The model under review builds one solid part; all positions refer to its coordinate system, in mm. A direction names the side the tool comes from. Round coordinates to 2 decimals unless told otherwise and drop trailing zeros. Write each loop counter-clockwise with the first axis right and the second up, starting at its lowest first coordinate (ties: lowest second). Pieces come first, ordered by that corner, then holes. Notation, with made-up numbers: M 12,-9 L 29,-9 A21 cw 29,23 Z; hole C -31.5,-4.5 d2. An arc over 180 degrees is marked long. Write item = value, one per line. Start each with the question number.
Item 1: Tool access review of faces 1 (the flat face through (-62, 40, -1)), 2 (the flat face through (-88, 20, 1)): name each direction out of +Z, -Z, +X, -X, +Y, -Y from which nothing blocks a thin tool from reaching the whole face with its end or side.
Item 2: The part is to be moulded in two halves that separate along Z. For faces 3 (the flat face through (28.5, 20, -136)), 4 (the flat face through (-205, 20, 2)), say which applies: +Z half, -Z half, draft (parallel to the pull), parting line (faces both ways), or undercut.
Item 3: Take a section at A-A, the plane x = 74. Give the boundary of the cut face in (y, z).
Item 4: Take a section at B-B, the plane z = 97.5. Give the boundary of the cut face in (x, y).
Item 5: Take a section at D-D, the plane x = 14. Give the boundary of the cut face in (y, z).
Item 6: Take a section at C-C, the plane y = 29. Give the boundary of the cut face in (x, z).
Item 7: To check wall thickness, follow line 1 along X through (y, z) = (16.5, -73); line 2 along Z through (x, y) = (-3.5, 17); line 3 along Z through (x, y) = (-116, 22). State the ranges of each line that lie inside material, in increasing order.
from build123d import *

# Parameters (mm, degrees)
SKETCH1_W           = 410
SKETCH1_H           = 341
BOSS_EXTRUDE1_DEPTH = 40


with BuildPart() as part:
    # Sketch1 → Boss-Extrude1 (new body)
    with BuildSketch(Plane(origin=(0, 0, 0), x_dir=(1, 0, 0), z_dir=(0, 1, 0))):
        Rectangle(SKETCH1_W, SKETCH1_H)
        with BuildLine():
            Line((28.5, 131.5), (28.5, 141.5))
            ThreePointArc((28.5, 141.5), (29.964466094, 145.035533906), (33.5, 146.5))
            Line((33.5, 146.5), (93.5, 146.5))
            ThreePointArc((93.5, 146.5), (97.035533906, 145.035533906), (98.5, 141.5))
            Line((98.5, 141.5), (98.5, 131.5))
            Line((98.5, 131.5), (180, 131.5))
            Line((180, 131.5), (180, -131.5))
            Line((180, -131.5), (98.5, -131.5))
            Line((98.5, -131.5), (98.5, -141.5))
            ThreePointArc((98.5, -141.5), (97.035533906, -145.035533906), (93.5, -146.5))
            Line((93.5, -146.5), (33.5, -146.5))
            ThreePointArc((33.5, -146.5), (29.964466094, -145.035533906), (28.5, -141.5))
            Line((28.5, -141.5), (28.5, -131.5))
            Line((28.5, -131.5), (-53, -131.5))
            Line((-53, -131.5), (-53, 131.5))
            Line((-53, 131.5), (28.5, 131.5))
        make_face(mode=Mode.SUBTRACT)
        Polygon((-184, -116.5), (-98, -116.5), (-88, -106.5), (-88, 106.5), (-98, 116.5), (-184, 116.5), align=None, mode=Mode.SUBTRACT)
    extrude(amount=BOSS_EXTRUDE1_DEPTH)


solid = part.part
Response values:
q1.face_1 = +Z, -Z, +X, -X, +Y
q1.face_2 = +Y, -Y
q2.face_3 = undercut
q2.face_4 = draft
q3.outline = M 0,-170.5 L 40,-170.5 L 40,-146.5 L 0,-146.5 Z; M 0,146.5 L 40,146.5 L 40,170.5 L 0,170.5 Z
q4.outline = M -205,0 L -184,0 L -184,40 L -205,40 Z; M -88,0 L -53,0 L -53,40 L -88,40 Z; M 180,0 L 205,0 L 205,40 L 180,40 Z
q5.outline = M 0,-170.5 L 40,-170.5 L 40,-131.5 L 0,-131.5 Z; M 0,131.5 L 40,131.5 L 40,170.5 L 0,170.5 Z
q6.outline = M -205,-170.5 L 205,-170.5 L 205,170.5 L -205,170.5 Z; hole M -184,-116.5 L -98,-116.5 L -88,-106.5 L -88,106.5 L -98,116.5 L -184,116.5 Z; hole M -53,-131.5 L 28.5,-131.5 L 28.5,-141.5 A5 ccw 33.5,-146.5 L 93.5,-146.5 A5 ccw 98.5,-141.5 L 98.5,-131.5 L 180,-131.5 L 180,131.5 L 98.5,131.5 L 98.5,141.5 A5 ccw 93.5,146.5 L 33.5,146.5 A5 ccw 28.5,141.5 L 28.5,131.5 L -53,131.5 Z
q7.line_1 = -205 to -184, -88 to -53, 180 to 205
q7.line_2 = -170.5 to -131.5, 131.5 to 170.5
q7.line_3 = -170.5 to -116.5, 116.5 to 170.5
